Geometry check sheet. Reference: the model listing, model coordinates, mm. A direction names the side the tool comes from. Give positions to 0.01 mm unless a question says otherwise; leave off trailing zeros. Loops run counter-clockwise (first coordinate to the right, second up) from the corner with the lowest first, then second, coordinate; pieces in that order, holes last. Notation, with made-up numbers: (86.5, 34) -> (126.5, 34) arc R24 cw to (126.5, 62) -> close; hole circle Ø11 at (6, -37.5). An arc over 180 degrees is marked (long way). Write item = value, one per line.
Autodesk Inventor part; units mm, degrees
ref_plane "YZ Plane" through (0, 0, 0) normal (1, 0, 0) x (0, 1, 0)
ref_plane "XZ Plane" through (0, 0, 0) normal (0, 1, 0) x (-1, 0, 0)
ref_plane "XY Plane" through (0, 0, 0) normal (0, 0, 1) x (1, 0, 0)
ref_plane "Work Plane1" through (0, 0, 0) normal (0, 0, 1) x (1, 0, 0)
sketch "Sketch1" plane through (0, 0, 0) normal (0, 0, 1) x (1, 0, 0)
  circle A0 centre (0, 0) radius 78.5
  line L0 (0, 0) -> (103.944697, 103.944697)
  line L1 (0, 0) -> (147, 0) construction
  line L2 (103.944697, 103.944697) -> (102.17693, 105.712464)
  line L3 (103.944697, 103.944697) -> (105.679378, 102.270109)
  circle A1 centre (0, 0) radius 71
  line L4 (105.742236, 95.137281) -> (55.226256, 44.621302)
  line L5 (109.340638, 98.735683) -> (180.781021, 98.735683) construction
  line L6 (95.105862, 105.712464) -> (44.620391, 55.226993)
  line L7 (98.641396, 109.247998) -> (170.038634, 109.247998) construction
  line L8 (44.257728, 44.257728) -> (66.757728, 44.257728)
  line L9 (66.757728, 44.257728) -> (66.757728, 66.757728)
  line L10 (66.757728, 66.757728) -> (44.257728, 66.757728)
  line L11 (44.257728, 66.757728) -> (44.257728, 44.257728)
  line L12 (44.257728, 44.257728) -> (66.757728, 66.757728) construction
  line L13 (66.757728, 44.257728) -> (44.257728, 66.757728) construction
  arc A2 (102.17693, 105.712464) -> (95.105862, 105.712464) centre (98.641396, 102.17693) ccw
  arc A3 (105.742236, 95.137281) -> (105.679378, 102.270109) centre (102.206702, 98.672815) ccw
  line L14 (44.257728, 66.757728) -> (35.912715, 61.247669)
  line L15 (66.757728, 44.257728) -> (61.247669, 35.912715)
  point P0 (55.507728, 55.507728)
  point P1 (55.518047, 44.257728)
  point P2 (66.757728, 56.152774)
  point P3 (56.151126, 66.757728)
  point P4 (44.257728, 55.518047)
  dimension "d0" = 157
  dimension "d1" = 147
  dimension "d2" = 45
  dimension "d3" = 7.5
  dimension "d4" = 7.5
  dimension "d5" = 142
  dimension "d6" = 135
  dimension "d7" = 135
  dimension "d8" = 22.5
  dimension "d9" = 22.5
  dimension "d10" = 5
  dimension "d34" = 10
  dimension "d35" = 10
extrude "Extrusion1" add sketch "Sketch1" along normal blind 2 contours L15 A1 L8 A0 | A0 L8 L15 | L14 L11 A0 | A0 L11 A1 L14 | L8 A1 L4 A0 | A0 L4 L9 L8 | L11 L10 L6 A0 | A0 L6 A1 L11 | L4 A1 L0 A0 | A0 L0 L9 L4 | L9 L0 L3 A3 L4 | L6 L10 L0 A0 | A0 L0 A1 L6 | L6 A2 L2 L0 L10
sketch "Sketch2" plane through (0, 0, 2) normal (0, 0, 1) x (1, 0, 0)
  circle A0 centre (0, 0) radius 78.5
  circle A1 centre (0, 0) radius 71
  line L0 (105.679378, 102.270109) -> (103.944697, 103.944697)
  line L1 (103.944697, 103.944697) -> (61.51829, 61.51829)
  line L2 (103.944697, 103.944697) -> (163.944697, 103.944697) construction
  line L3 (103.944697, 103.944697) -> (102.17693, 105.712464)
  line L4 (44.257728, 66.757728) -> (44.257728, 55.518047)
  line L5 (55.518047, 44.257728) -> (66.757728, 44.257728)
  line L6 (46.257728, 66.757728) -> (46.257728, 55.518047)
  line L7 (55.518047, 46.257728) -> (66.757728, 46.257728)
  line L8 (61.51829, 61.51829) -> (60.113782, 62.942143)
  line L9 (60.113782, 62.942143) -> (62.922798, 60.094437)
  arc A2 (105.742236, 95.137281) -> (105.679378, 102.270109) centre (102.206702, 98.672815) ccw
  line L10 (62.922798, 60.094437) -> (105.679378, 102.270109)
  line L11 (60.113782, 62.942143) -> (102.530516, 105.358877)
  line L12 (60.113782, 62.942143) -> (120.100103, 62.942143) construction
  line L13 (46.257728, 55.518047) -> (46.257728, 53.862998)
  line L14 (55.518047, 46.257728) -> (53.862998, 46.257728)
  line L15 (56.151126, 66.757728) -> (44.257728, 66.757728)
  line L16 (44.257728, 66.757728) -> (35.912715, 61.247669)
  line L17 (66.757728, 44.257728) -> (61.247669, 35.912715)
  point P0 (58.399252, 46.257728)
  point P1 (63.422966, 46.257728)
  point P2 (46.257728, 63.422966)
  point P3 (46.257728, 58.399252)
  point P4 (44.257728, 64.834432)
  point P5 (64.834432, 44.257728)
  point P6 (65.800574, 42.808113)
  point P7 (42.808113, 65.800574)
  dimension "d13" = 157
  dimension "d14" = 7.5
  dimension "d16" = 135
  dimension "d21" = 2
  dimension "d22" = 2
  dimension "d25" = 60
  dimension "d26" = 2
  dimension "d27" = 4
  dimension "d28" = 45
  dimension "d32" = 10
  dimension "d33" = 10
extrude "Extrusion2" add sketch "Sketch2" along normal blind 22 contours L17 A1 L5 A0 | A0 L4 A1 L16 | L5 A1 L14 L7 A0 | A0 L6 L13 A1 L4 | L7 L14 A1 L13 L6 A0 | L10 L9 L1 L0 | L1 L8 L11 L3
chamfer "Chamfer1" distance 2 angle 45 3 edges at (84.3011, 81.1823, 2) (81.3221, 84.1505, 2) (61.5183, 61.5183, 2)
chamfer "Chamfer2" distance 5 angle 45 3 edges at (66.7577, 56.1528, 1) (56.1511, 66.7577, 1) (61.5183, 61.5183, 24)
properties part number "HourGuard"
Item 1: Gauge pin test, flat ends, axial feed: pin 1 (1.6 mm diameter, centred on y = 47.5, z = 1.5, fed in from +X); pin 2 (1.5 mm diameter, centred on x = 91, z = 19.5, fed in from -Y); pin 3 (5 mm diameter, centred on x = 75, z = 16.5, fed in from -Y). Record the tip position at first contact, or that the pin passes through.
Answer:
pin_1 = 66.76
pin_2 = 87.05
pin_3 = 69.54
Item 2: Tool access check on faces 4 (the flat face through (66.758, 48, 1)), 5 (the flat face through (53, 52, 24)), 6 (the flat face through (104.8, 103.12, 11.83)), 7 (the flat face through (48, 66.758, 1)), 8 (the flat face through (63.241, 63.282, 21.465)). Record the directions out of +Z, -Z, +X, -X, +Y, -Y that give a thin tool (end or side, any length) a straight path to the whole face; none if there is none.
Answer:
face_4 = +Z, -Z, +X, -Y
face_5 = +Z, +X, -X, +Y, -Y
face_6 = +Z, -Z, +X, +Y
face_7 = +Z, -Z, -X, +Y
face_8 = +Z
Item 3: Section check A-A, the plane z = 8.5. Record the cut outline in (x, y).
Answer:
outline = (35.91, 61.25) arc R71 cw to (61.25, 35.91) -> (65.8, 42.81) arc R78.5 ccw to (42.81, 65.8) -> close; (60.11, 62.94) -> (62.92, 60.09) -> (105.68, 102.27) -> (103.94, 103.94) -> (102.53, 105.36) -> close
Item 4: Draft check along X on faces 1 (the flat face through (103.27, 104.62, 11.83)), 2 (the flat face through (77, 70, 2)), 3 (the flat face through (85, 85, 24)). Enter one of: +X half, -X half, draft (parallel to the pull), parting line (faces both ways), or undercut.
Answer:
face_1 = +X half
face_2 = undercut
face_3 = draft
Item 5: Thickness scan on L1, parallel to X at y = 64.5, z = 20.75; L2, parallel to Y at x = 60.5, z = 18.25; L3, parallel to Z at x = 76, y = 84. Record the ranges inside material, lowest first. Write a range as [from, to].
Answer:
L1 = [40.84, 44.74], [61.67, 67.39]
L2 = [37.16, 50.02], [62.55, 63.33]
L3 = [0, 2]
Item 6: Section check C-C, the plane x = 99.5. Record the cut outline in (y, z), plus the area to 3 significant figures.
Answer:
outline = (88.9, 0) -> (107.1, 0) -> (107.1, 2) -> (105.16, 2) -> (102.33, 4) -> (102.33, 24) -> (96.17, 24) -> (96.17, 4) -> (93.37, 2) -> (88.9, 2) -> close
area = 177 mm^2
Item 7: Section check B-B, the plane y = 79.5. Record the cut outline in (x, z).
Answer:
outline = (68.89, 0) -> (90.1, 0) -> (90.1, 2) -> (85.44, 2) -> (82.6, 4) -> (82.6, 24) -> (76.67, 24) -> (76.67, 4) -> (73.84, 2) -> (68.89, 2) -> close
